The listing builds one solid part. Answer for the finished solid, in the listing's coordinates (mm). Coordinates: 2 decimals unless noted, no trailing zeros. Loops run counter-clockwise (first coordinate to the right, second up) from the corner with the lowest first, then second, coordinate; pieces in that order, holes last. Notation, with made-up numbers: M 41.5,38.5 L 58.5,38.5 A5 ccw 58.5,47.5 Z; hole C 38.25,41.25 d9. An arc over 180 degrees is marked long. Answer in a Markdown table with one row per item. Add a question column.
from build123d import *

# Parameters (mm, degrees)
BASPROSKE_W     = 10
BASPROSKE_H     = 7
TOOTHCUT_DEPTH  = 15.071247279
TEETHCUTS_COUNT = 12
TEETHCUTS_ANGLE = 330
BORSKE_R        = 2
BORE_DEPTH      = 50.0000508
CHAMFER_1_SIZE  = 2


with BuildPart() as part:
    # BasProSke → Base-Revolve (revolve)
    with BuildSketch(Plane(origin=(0, 0, 0), x_dir=(1, 0, 0), z_dir=(0, 1, 0)), mode=Mode.PRIVATE) as base_revolve_sk:
        with Locations((5, 3.5)):
            Rectangle(BASPROSKE_W, BASPROSKE_H)
    revolve(base_revolve_sk.sketch.rotate(Axis((-10, 0, 0), (1, 0, 0)), 180), axis=Axis((-10, 0, 0), (1, 0, 0)))

    # TooCutSke → ToothCut (cut, through all)
    with BuildSketch(Plane(origin=(0, 0, 0), x_dir=(0, 0, -1), z_dir=(1, 0, 0))):
        with BuildLine():
            ThreePointArc((0.562207301, 4.715604304), (0, 4.749), (-0.562207301, 4.715604304))
            ThreePointArc((-0.562207301, 4.715604304), (-0.837528627, 5.917009812), (-1.672850686, 6.823328788))
            ThreePointArc((-1.672850686, 6.823328788), (0, 7.0254), (1.672850686, 6.823328788))
            ThreePointArc((1.672850686, 6.823328788), (0.837528627, 5.917009812), (0.562207301, 4.715604304))
        make_face()
    toothcut = extrude(amount=TOOTHCUT_DEPTH, mode=Mode.SUBTRACT)

    # TeethCuts: ToothCut ×12 about axis
    teethcuts_axis = Axis((-10, 0, 0), (1, 0, 0))
    for i in range(1, TEETHCUTS_COUNT):
        add(toothcut.rotate(teethcuts_axis, i * TEETHCUTS_ANGLE / (TEETHCUTS_COUNT - 1)), mode=Mode.SUBTRACT)

    # BorSke → Bore (cut, symmetric)
    with BuildSketch(Plane(origin=(0, 0, 0), x_dir=(0, 0, -1), z_dir=(1, 0, 0))):
        with Locations(Location((0, 0, 0), (0, 0, 180))):
            Circle(BORSKE_R)
    extrude(amount=BORE_DEPTH, both=True, mode=Mode.SUBTRACT)

    # 倒角1
    chamfer_1_edges = [part.edges().sort_by_distance(p)[0] for p in [
        (0, 0, -2),
    ]]
    chamfer(chamfer_1_edges, length=CHAMFER_1_SIZE)


solid = part.part
(1) A cutting plane is placed at A-A (z = 0). Give the vertices of the cut face in (x, y).
(2) Each of these flat-tipped pins is pushed along its axis until it touches: pin 1 (5 mm diameter, centred on x = 5.5, y = 0.5, fed in from -Z); pin 2 (5 mm diameter, centred on x = 2.5, z = 0, fed in from -Y); pin 3 (4.5 mm diameter, centred on y = 0, z = 0, fed in from -X). Where does it stop, or does it pass through?
(3) Straight lines are drawn through the part: line 1 (Z direction, x = 7.5, y = -4.5); line 2 (Y direction, x = 8.25, z = -4); line 3 (Y direction, x = 3.25, z = 6). For each, find the intervals that lie inside material, in ascending order.
(4) The mould has two halves that part along Y. Classify faces 1 (the face through (0, -4, -2)), 2 (the face through (4.93, 3.684, 4.705)): released by +Y, released by -Y, zero draft, split by the parting line, or undercut.
Solved:
| question | item | result |
|---|---|---|
| 1 | outline | M 0,-4.75 L 10,-4.75 L 10,-2 L 2,-2 L 0,-4 Z; M 0,4 L 2,2 L 10,2 L 10,4.75 L 0,4.75 Z |
| 2 | pin 1 | stops at z = -6.8 |
| 2 | pin 2 | stops at y = -6.8 |
| 2 | pin 3 | stops at x = 1.75 |
| 3 | line 1 | z = -5.03 to -3.4, -1.95 to 1.95, 3.4 to 5.03 |
| 3 | line 2 | y = -4.87 to -2.96, -2.56 to 2.56, 2.96 to 4.87 |
| 3 | line 3 | y = -2.21 to -0.88, 0.88 to 2.21 |
| 4 | face 1 | zero draft |
| 4 | face 2 | undercut |
